Work out the finished part from the listing and answer in its coordinate system (mm). A direction names the side the tool comes from. Round coordinates to 2 decimals unless told otherwise and drop trailing zeros. Order: outer loops, then holes, each group sorted by start corner. A loop starts at its lowest first (then second) coordinate and runs counter-clockwise, first axis right, second up. Notation, with made-up numbers: (83, 47.25) -> (101, 47.25) arc R8 cw to (101, 59.25) -> close; hole circle Ø8 at (37.5, 58). An arc over 180 degrees is marked (long way). Use one line per item in the form item = value.
Autodesk Inventor part; units mm, degrees
ref_plane "YZ Plane" through (0, 0, 0) normal (1, 0, 0) x (0, 1, 0)
ref_plane "XZ Plane" through (0, 0, 0) normal (0, 1, 0) x (-1, 0, 0)
ref_plane "XY Plane" through (0, 0, 0) normal (0, 0, 1) x (1, 0, 0)
sketch "Sketch1" plane through (0, 0, 0) normal (0, 1, 0) x (-1, 0, 0)
  circle A0 centre (0, 0) radius 4.875
  dimension "d0" = 9.75
extrude "Extrusion1" add sketch "Sketch1" along normal blind 10
sketch "Sketch2" plane through (0, 0, 0) normal (1, 0, 0) x (0, 1, 0)
  line L0 (0, 0) -> (10, 0)
  line L1 (10, -4.875) -> (10, 4.875)
  line L2 (10, 0) -> (10, -6.5)
  arc A0 (10, -6.5) -> (12.3658, 0) centre (-5.6698, 2.8839) ccw
  line L3 (10, -6.5) -> (12.3658, 0) construction
  line L4 (10, -6.5) -> (16.9172, -6.5) construction
  line L5 (0, -4.875) -> (10, -4.875)
  arc A1 (8.6365, -4.875) -> (10, -6.5) centre (10.6414, -4.5773) ccw
  line L6 (10, -6.5) -> (8.6365, -4.875) construction
  line L7 (10, -6.5) -> (12.1213, -6.5) construction
  line L8 (8.6365, -4.875) -> (8.6365, 0)
  line L9 (12.3658, 0) -> (8.6365, 0)
  line L10 (12.3658, 0) -> (0, 0)
  line L11 (0, -4.875) -> (0, 4.875)
  dimension "d8" = 6.5
  dimension "d9" = 70
  dimension "d10" = 130
revolve "Revolution1" add sketch "Sketch2" angle 360 about axis through (0, 0, 0) along (0, 1, 0) contours L9 A0 L2 L1 | L5 L2 A1
sketch "Sketch4" plane through (0, 0, 0) normal (0, -1, 0) x (1, 0, 0)
  circle A0 centre (0, 0) radius 2
  dimension "d11" = 4
extrude "Extrusion2" cut sketch "Sketch4" against normal through all
fillet "Fillet2" radius 0.5 5 edges at (0, 10, 6.5) (1.4142, 11.9298, -1.4142) (-1.4141, 11.9298, 1.4143) (-3.4471, 8.6365, -3.4471) (3.4471, 8.6365, 3.4471)
properties part number "Part3pasador"
Item 1: The part is cut by section A-A, the plane y = 6.25. Give the vertices of the cut face in (x, z) (3 decimals).
Findings:
outline = circle Ø9.75 at (0, 0); hole circle Ø4 at (0, 0)
Item 2: Flat-ended cylindrical pins translate along their axes: P1, Ø2, axis at x = 2, z = 4, coming from the +Y side; P2, Ø4, axis at y = 6, z = -2, coming from the -X side (3 decimals); P3, Ø6, axis at x = -1, y = 2, coming from the -Z side (3 decimals); P4, Ø1.5, axis at x = -3.5, z = -2.5, coming from the -Y side. Find the tip coordinate at first contact, or state that the pin passes through.
Findings:
P1 = 11.45
P2 = -4.875
P3 = -4.875
P4 = 0
Item 3: Consider line 1 along Z through (x, y) = (0, 3) (3 decimals); line 2 along Y through (x, z) = (2, 1.75). Determine where each line is inside the solid, lowest interval first.
Findings:
line_1 = -4.875 to -2, 2 to 4.875
line_2 = 0 to 11.73
Item 4: For faces 1 (the cylindrical face through (0.635, 4.064, -4.834)), 2 (the flat face through (-2, 0, -1)), determine the directions among +Z, -Z, +X, -X, +Y, -Y from which every point of the face is accessible in a straight line to the end or side of a thin tool.
Findings:
face_1 = -Y
face_2 = +Z, -Z, +X, -X, -Y
